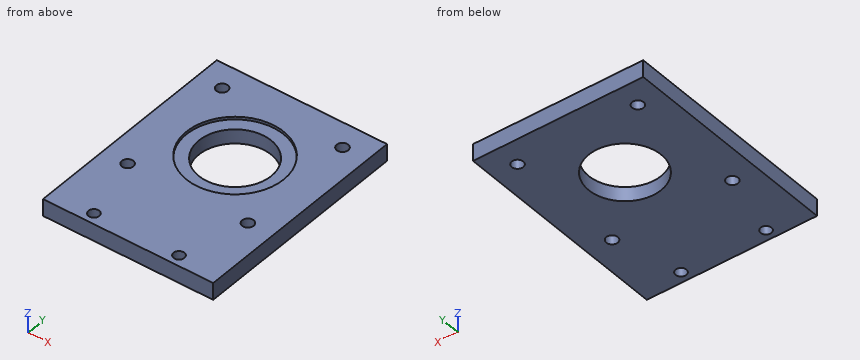
Autodesk Inventor part; units mm, degrees
ref_plane "YZ Plane" through (0, 0, 0) normal (1, 0, 0) x (0, 1, 0)
ref_plane "XZ Plane" through (0, 0, 0) normal (0, 1, 0) x (-1, 0, 0)
ref_plane "XY Plane" through (0, 0, 0) normal (0, 0, 1) x (1, 0, 0)
sketch "Sketch1" plane through (0, 0, 0) normal (0, 0, 1) x (1, 0, 0)
  line L0 (0, 0) -> (200, 0)
  line L1 (200, 0) -> (200, 260)
  line L2 (200, 260) -> (0, 260)
  line L3 (0, 260) -> (0, 0)
  dimension "d0" = 200
  dimension "d1" = 260
extrude "Extrusion1" add sketch "Sketch1" along normal blind 20
sketch "Sketch2" plane through (0, 0, 20) normal (0, 0, 1) x (1, 0, 0)
  circle A0 centre (100, 160) radius 42.5
  line L0 (200, 260) -> (0, 260)
  line L1 (0, 260) -> (0, 0)
  dimension "d4" = 85
  dimension "d5" = 100
  dimension "d6" = 100
extrude "Extrusion2" cut sketch "Sketch2" against normal blind 30
sketch "Sketch6" plane through (0, 0, 0) normal (0, 0, -1) x (-1, 0, 0)
  circle A0 centre (-29.289, 230.711) radius 6.75
  circle A1 centre (-170.711, 230.711) radius 6.75
  circle A2 centre (-170.711, 89.289) radius 6.75
  circle A3 centre (-29.289, 89.289) radius 6.75
  circle A4 centre (-100, 160) radius 42.5
  circle A5 centre (-50.0126, 12.4968) radius 6.35
  circle A6 centre (-149.9874, 12.4968) radius 6.35
  line L0 (-200, 0) -> (-200, 260)
  line L1 (0, 260) -> (0, 0)
  line L2 (0, 0) -> (-200, 0)
  dimension "d18" = 70.711
  dimension "d19" = 70.711
  dimension "d20" = 70.711
  dimension "d21" = 70.711
  dimension "d22" = 70.711
  dimension "d23" = 70.711
  dimension "d24" = 70.711
  dimension "d25" = 70.711
  dimension "d26" = 13.5
  dimension "d27" = 13.5
  dimension "d28" = 13.5
  dimension "d29" = 13.5
  dimension "d57" = 12.7
  dimension "d58" = 12.7
  dimension "d59" = 50.0126
  dimension "d60" = 50.0126
  dimension "d61" = 12.4968
  dimension "d62" = 12.4968
extrude "Extrusion6" cut sketch "Sketch6" against normal blind 20 contours A0 | A1 | A2 | A3 | A5 | A6
sketch "Sketch12" plane through (0, 0, 20) normal (0, 0, 1) x (1, 0, 0)
  circle A0 centre (100, 160) radius 42.5
  circle A1 centre (100, 160) radius 57.15
  point P0 (0, 0)
  dimension "d66" = 114.3
extrude "Extrusion11" cut sketch "Sketch12" against normal blind 3.2 contours A0 | A1
equation "\"d19\" = d18"
equation "\"d20\" = d18"
equation "\"d21\" = d19"
equation "\"d22\" = d20"
equation "\"d23\" = d22"
equation "\"d24\" = d23"
equation "\"d25\" = d23"
equation "\"d58\" = d57"
properties part number "FloorMount"
Read the model definition and answer for the solid it produces. Units are mm, in the model's axes. Give positions to 0.01 mm unless a question says otherwise; leave off trailing zeros. Loops run counter-clockwise (first coordinate to the right, second up) from the corner with the lowest first, then second, coordinate; pieces in that order, holes last. Notation, with made-up numbers: (13, 59) - (68, 59) arc R30 cw to (68, 89) - close; hole circle Ø5 at (41.5, 72.5). An arc over 180 degrees is marked (long way). Answer as CSV lines item,"result". Start each with the question number.
1) Find section D-D (y = 92). Write down the section's boundary in (x, z).
2) Find section B-B (y = 160). Write down the section's boundary in (x, z), then the cut area to 3 significant figures.
3) Straight lines are drawn through the part: L1, parallel to X at y = 225.5, z = 13.5; L2, parallel to Y at x = 26.5, z = 17.5; L3, parallel to Z at x = 120.5, y = 204.5. For each, find the intervals that lie inside material, in ascending order. Write a range as from..to.
4) Find section C-C (z = 12.5). Write down the section's boundary in (x, y), then the cut area to 3 significant figures.
5) This flat-tipped pin is pushed along its axis until it touches: pin 1 Ø4 at (y, z) = (171.5, 4.5) entering from -X. Where does it stop, or does it pass through?
6) Find section A-A (x = 100). Write down the section's boundary in (y, z), then the cut area to 3 significant figures.
Findings below:
1,outline,"(0, 0) - (23.11, 0) - (23.11, 20) - (0, 20) - close; (35.47, 0) - (164.53, 0) - (164.53, 20) - (35.47, 20) - close; (176.89, 0) - (200, 0) - (200, 20) - (176.89, 20) - close"
2,outline,"(0, 0) - (57.5, 0) - (57.5, 16.8) - (42.85, 16.8) - (42.85, 20) - (0, 20) - close; (142.5, 0) - (200, 0) - (200, 20) - (157.15, 20) - (157.15, 16.8) - (142.5, 16.8) - close"
2,area,"2,210 mm^2"
3,L1,"0..25, 33.58..166.42, 175..200"
3,L2,"0..83.14, 95.44..224.56, 236.86..260"
3,L3,"0..16.8"
4,outline,"(0, 0) - (200, 0) - (200, 260) - (0, 260) - close; hole circle Ø13.5 at (29.29, 89.29); hole circle Ø13.5 at (29.29, 230.71); hole circle Ø12.7 at (50.01, 12.5); hole circle Ø85 at (100, 160); hole circle Ø12.7 at (149.99, 12.5); hole circle Ø13.5 at (170.71, 89.29); hole circle Ø13.5 at (170.71, 230.71)"
4,area,"45,500 mm^2"
5,pin 1,"x = 0"
6,outline,"(0, 0) - (117.5, 0) - (117.5, 16.8) - (102.85, 16.8) - (102.85, 20) - (0, 20) - close; (202.5, 0) - (260, 0) - (260, 20) - (217.15, 20) - (217.15, 16.8) - (202.5, 16.8) - close"
6,area,"3,410 mm^2"
